Geometry check sheet. Reference: drawing and pictorial views, mm from the part's lowest x, y, z. A direction names the side the tool comes from. Give positions to 0.01 mm unless a question says otherwise; leave off trailing zeros. Write each loop counter-clockwise with the first axis right and the second up, starting at its lowest first coordinate (ties: lowest second). Pieces come first, ordered by that corner, then holes. Notation, with made-up numbers: (42, 24) - (70, 24) arc R14 cw to (70, 30) - close; hole circle Ø1 at (19, 62). An arc over 180 degrees is marked (long way). Put each result on its own line as item: value.
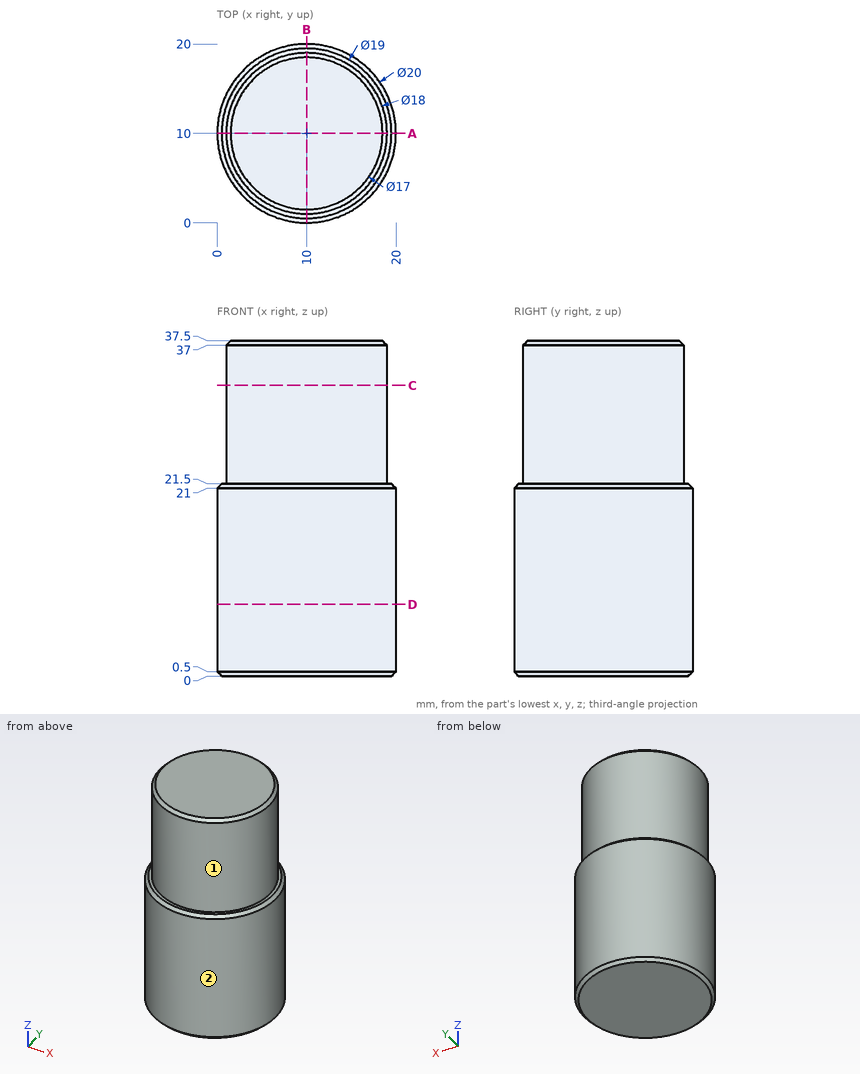
Q1. Section check A-A, the plane y = 10. Record the cut outline in (x, z), plus the area to 3 significant figures.
Answers follow:
outline: (0, 0.5) - (0.5, 0) - (19.5, 0) - (20, 0.5) - (20, 21) - (19.5, 21.5) - (19, 21.5) - (19, 37) - (18.5, 37.5) - (1.5, 37.5) - (1, 37) - (1, 21.5) - (0.5, 21.5) - (0, 21) - close
area: 717 mm2
Q2. Scan lines: line 1 along X through (y, z) = (4.75, 15.5); line 2 along Z through (x, y) = (19.25, 9.75); line 3 along X through (y, z) = (8.5, 24). Record each from-to range of solid material in increasing order.
Answers follow:
line 1: x = 1.49 to 18.51
line 2: z = 0 to 21.5
line 3: x = 1.13 to 18.87
Q3. Section check C-C, the plane z = 32.5. Record the cut outline in (x, y), plus the area to 3 significant figures.
Answers follow:
outline: circle Ø18 at (10, 10)
area: 254 mm2
Q4. Go/stop test with flat-tipped pins: pin 1 Ø6 at (x, z) = (14, 27) entering from +Y; pin 2 Ø1.5 at (x, z) = (5.5, 11) entering from -Y; pin 3 Ø1 at (x, y) = (11, 17) entering from -Z; pin 4 Ø6 at (y, z) = (3.5, 28.5) entering from -X. Record where each tip stops, or that it passes through.
Answers follow:
pin 1: stops at y = 18.94
pin 2: stops at y = 0.73
pin 3: stops at z = 0
pin 4: stops at x = 1.71
Q5. Section check D-D, the plane z = 8. Record the cut outline in (x, y), plus the area to 3 significant figures.
Answers follow:
outline: circle Ø20 at (10, 10)
area: 314 mm2
Q6. Set-up check for the marked faces 1 and 2: record each of +Z, -Z, +X, -X, +Y, -Y from which the full face is reachable in a straight line by a thin tool's end or side.
Answers follow:
face 1: +Z
face 2: +Z, -Z
